Study the drawing (mm; zero at the part's minimum x, y, z) and answer. A direction names the side the tool comes from. Give positions to 0.01 mm unless a question says otherwise; leave off trailing zeros. Write each loop counter-clockwise with the first axis right and the second up, starting at its lowest first coordinate (ties: lowest second). Pieces come first, ordered by that corner, then holes. Notation, with made-up numbers: (59, 31) - (102, 31) arc R29 ccw to (102, 51) - close; hole circle Ø4 at (48, 31.25). An arc over 180 degrees is marked (long way). One line per item, written item: value. Start each with the question number.
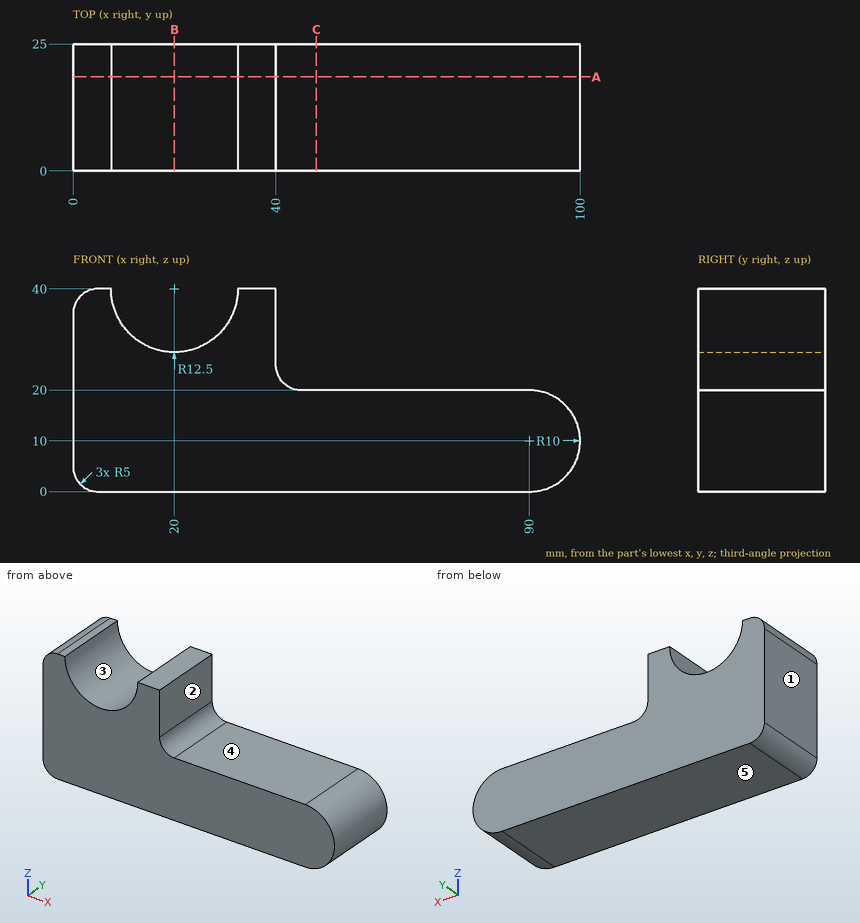
Item 1: Find section B-B on x = 20. Determine the outline of the cut face in (y, z), plus the area to 4 significant figures.
Item 2: The mould has two halves that part along X. Classify the marked faces 1, 2 and 3: +X half, -X half, draft (parallel to the pull), parting line (faces both ways), or undercut.
Item 3: For the marked faces 4 and 5, determine the directions among +Z, -Z, +X, -X, +Y, -Y from which every point of the face is accessible in a straight line to the end or side of a thin tool.
Item 4: Each of these flat-tipped pins is pushed along its axis until it touches: pin 1 Ø4 at (x, y) = (59.5, 19) entering from +Z; pin 2 Ø6 at (y, z) = (16, 33) entering from +X; pin 3 Ø5 at (y, z) = (7, 4.5) entering from -X. Where does it stop, or does it pass through?
Item 5: Find section C-C on x = 48. Determine the outline of the cut face in (y, z).
Item 6: Find section A-A on y = 18.5. Determine the outline of the cut face in (x, z), plus the area to 3 significant figures.
Item 7: Straight lines are drawn through the part: line 1 along Z through (x, y) = (62, 13); line 2 along X through (y, z) = (19.25, 27); line 3 along X through (y, z) = (23, 38). For each, find the intervals that lie inside material, in ascending order.
Values:
1. outline: (0, 0) - (25, 0) - (25, 27.5) - (0, 27.5) - close
1. area: 687.5 mm^2
2. face 1: -X half
2. face 2: +X half
2. face 3: undercut
3. face 4: +Z, +X, +Y, -Y
3. face 5: -Z, +X, -X, +Y, -Y
4. pin 1: z = 20
4. pin 2: x = 40
4. pin 3: x = 0
5. outline: (0, 0) - (25, 0) - (25, 20) - (0, 20) - close
6. outline: (0, 5) arc R5 ccw to (5, 0) - (90, 0) arc R10 ccw to (90, 20) - (45, 20) arc R5 cw to (40, 25) - (40, 40) - (32.5, 40) arc R12.5 cw to (7.5, 40) - (5, 40) arc R5 ccw to (0, 35) - close
6. area: 2,510 mm^2
7. line 1: 0 to 20
7. line 2: 0 to 40
7. line 3: 1 to 7.66, 32.34 to 40
